Input: part model. Units: mm. Frame: model coordinates. Give positions to 0.01 mm unless a question says otherwise; leave off trailing zeros. Loops run counter-clockwise (first coordinate to the right, second up) from the corner with the lowest first, then second, coordinate; pieces in that order, holes last.
from build123d import *

# Parameters (mm, degrees)
SKETCH1_W           = 350
SKETCH1_H           = 50
BOSS_EXTRUDE1_DEPTH = 3
BOSS_EXTRUDE2_DEPTH = 350
SKETCH3_W           = 10.5
SKETCH3_H           = 6.5
CUT_EXTRUDE1_DEPTH  = 10


with BuildPart() as part:
    # Sketch1 → Boss-Extrude1 (new body)
    with BuildSketch(Plane(origin=(0, 0, 0), x_dir=(0, 1, 0), z_dir=(0, 0, 1))):
        Rectangle(SKETCH1_W, SKETCH1_H)
    extrude(amount=BOSS_EXTRUDE1_DEPTH)

    # Sketch2 → Boss-Extrude2 (add, through all)
    with BuildSketch(Plane.XZ.offset(175)):
        Polygon((-25, 3), (-25, 0), (-28, 0), align=None)
        Polygon((25, 3), (28, 0), (25, 0), align=None)
    extrude(amount=-BOSS_EXTRUDE2_DEPTH)

    # Sketch3 → Cut-Extrude1 (cut)
    with BuildSketch(Plane(origin=(0, 0, 0), x_dir=(1, 0, 0), z_dir=(0, 0, -1))):
        Polygon((0, 55), (10.5, 55), (10.5, 48.5), (-17, 48.5), (-17, 55), align=None)
        with Locations((0, -94.75)):
            Rectangle(SKETCH3_W, SKETCH3_H)
    extrude(amount=-CUT_EXTRUDE1_DEPTH, mode=Mode.SUBTRACT)


solid = part.part
(1) Ray query, probe 1 along Y at (x, z) = (3.5, 1.7); probe 2 along Y at (x, z) = (-6.5, 0.3); probe 3 along X at (y, z) = (28, 1.4). Return the intervals inside material, ascending.
Values follow:
probe 1: y = -175 to -55, -48.5 to 91.5, 98 to 175
probe 2: y = -175 to -55, -48.5 to 175
probe 3: x = -26.6 to 26.6
(2) Cut plane A-A (z = 1.9). Return the cut outline in (x, y).
Values follow:
outline: (-26.1, -175) - (26.1, -175) - (26.1, 175) - (-26.1, 175) - close; hole (-17, -55) - (10.5, -55) - (10.5, -48.5) - (-17, -48.5) - close; hole (-5.25, 91.5) - (5.25, 91.5) - (5.25, 98) - (-5.25, 98) - close
(3) Cut plane B-B (x = -1). Return the cut outline in (y, z), and give its area (3 significant figures).
Values follow:
outline: (-175, 0) - (-55, 0) - (-55, 3) - (-175, 3) - close; (-48.5, 0) - (91.5, 0) - (91.5, 3) - (-48.5, 3) - close; (98, 0) - (175, 0) - (175, 3) - (98, 3) - close
area: 1,010 mm2
(4) Cut plane C-C (y = 34). Return the cut outline in (x, z), and give its area (3 significant figures).
Values follow:
outline: (-28, 0) - (28, 0) - (25, 3) - (-25, 3) - close
area: 159 mm2
(5) Pin query (flat end, axial travel): pin 1 Ø1.5 at (x, y) = (17, -37) entering from -Z; pin 2 Ø0.9 at (y, z) = (95.5, 1) entering from -X; pin 3 Ø0.9 at (y, z) = (-53.5, 2) entering from +X; pin 4 Ø1.5 at (y, z) = (94.5, 2) entering from +X. Return the tip coordinate at first contact, or that it passes through.
Values follow:
pin 1: stops at z = 0
pin 2: stops at x = -27.45
pin 3: stops at x = 26.45
pin 4: stops at x = 26.75
